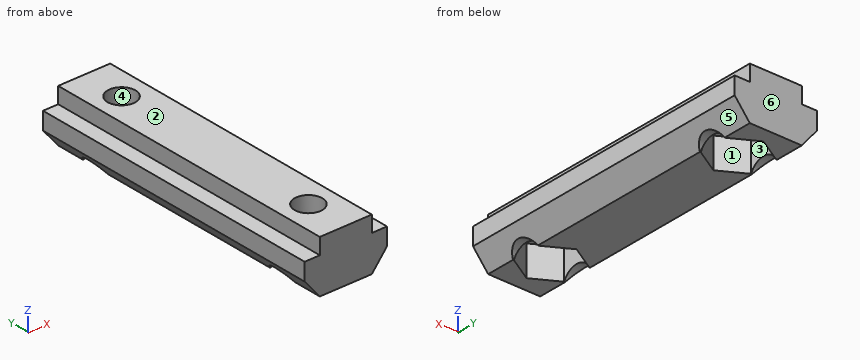
from build123d import *

# Parameters (mm, degrees)
EXTRUDE1_DEPTH = 35
EXTRUDE2_REACH = 8
SKETCH2_R      = 1.6
SKETCH_R       = 1.6
EXTRUDE3_DEPTH = 3.5
EXTRUDE4_START = -0.967619
EXTRUDE4_DEPTH = 7.735238


with BuildPart() as part:
    # Sketch1 → Extrude1 (new body)
    with BuildSketch(Plane(origin=(0, 0, 0), x_dir=(1, 0, 0), z_dir=(0, 1, 0))):
        Polygon((-3, 2.978553588), (3, 2.978553588), (3, 4.828553588), (4.75, 4.828553588), (4.75, 6.828553588), (3, 8.978553588), (-3, 8.978553588), (-4.75, 6.828553588), (-4.75, 4.828553588), (-3, 4.828553588), align=None)
    extrude(amount=EXTRUDE1_DEPTH)

    # Sketch2 → Extrude2 (cut, up to next)
    with BuildSketch(Plane(origin=(0, 0, -8.978553588), x_dir=(-1, 0, 0), z_dir=(0, 0, -1)), mode=Mode.PRIVATE) as extrude2_sk1:
        with Locations((0, 30)):
            Circle(SKETCH2_R)
    extrude2_tool1 = extrude(extrude2_sk1.sketch, amount=-EXTRUDE2_REACH, mode=Mode.PRIVATE) & part.part
    add(extrude2_tool1.solids().sort_by_distance((0, 30, -8.978554))[0], mode=Mode.SUBTRACT)
    # Sketch2 → Extrude2 (cut, up to next)
    with BuildSketch(Plane(origin=(0, 0, -8.978553588), x_dir=(-1, 0, 0), z_dir=(0, 0, -1)), mode=Mode.PRIVATE) as extrude2_sk2:
        with Locations((0, 5)):
            Circle(SKETCH2_R)
    extrude2_tool2 = extrude(extrude2_sk2.sketch, amount=-EXTRUDE2_REACH, mode=Mode.PRIVATE) & part.part
    add(extrude2_tool2.solids().sort_by_distance((0, 5, -8.978554))[0], mode=Mode.SUBTRACT)

    # Sketch → Extrude3 (cut)
    with BuildSketch(Plane(origin=(0, 0, -8.978553588), x_dir=(-1, 0, 0), z_dir=(0, 0, -1))):
        Polygon((0, 33.348631561), (-2.9, 31.674315781), (-2.9, 28.325684219), (0, 26.651368439), (2.9, 28.325684219), (2.9, 31.674315781), align=None)
        with Locations((0, 30)):
            Circle(SKETCH_R, mode=Mode.SUBTRACT)
        Polygon((2.9, 3.325684219), (0, 1.651368439), (-2.9, 3.325684219), (-2.9, 6.674315781), (0, 8.348631561), (2.9, 6.674315781), align=None)
        with Locations((0, 5)):
            Circle(SKETCH_R, mode=Mode.SUBTRACT)
    extrude(amount=-EXTRUDE3_DEPTH, mode=Mode.SUBTRACT)

    # Sketch3 → Extrude4 (cut)
    with BuildSketch(Plane(origin=(-2.9, 0, 0), x_dir=(0, 0, -1), z_dir=(1, 0, 0)).offset(EXTRUDE4_START)):
        with BuildLine():
            Line((8.978553588, 31.674315781), (8.978553588, 28.325684219))
            ThreePointArc((8.978553588, 28.325684219), (7.912621815, 30), (8.978553588, 31.674315781))
        make_face()
    extrude4 = extrude(amount=EXTRUDE4_DEPTH, mode=Mode.SUBTRACT)

    # Mirror1: Extrude4 across plane
    add(extrude4.mirror(Plane.ZX.offset(17.5)), mode=Mode.SUBTRACT)


solid = part.part
Part model, mm, in its own coordinate system. Face numbers are marked on the shaded views. A direction names the side the tool comes from. Give positions to 0.01 mm unless a question says otherwise; leave off trailing zeros. Order: outer loops, then holes, each group sorted by start corner. A loop starts at its lowest first (then second) coordinate and runs counter-clockwise, first axis right, second up. Notation, with made-up numbers: (45, -29) - (64, -29) arc R19 ccw to (64, 6) - close; hole circle Ø4 at (8, -36.75). An arc over 180 degrees is marked (long way). Use a Markdown table: item, result.
1) Saw through at B-B on z = -6.5. List the corners of the cut face in (x, y), plus the area to 3 significant figures.
Checked values:
| item | result |
|---|---|
| outline | (-4.75, 0) - (4.75, 0) - (4.75, 35) - (-4.75, 35) - close; hole (-2.9, 3.33) - (0, 1.65) - (2.9, 3.33) - (2.9, 6.67) - (0, 8.35) - (-2.9, 6.67) - close; hole (-2.9, 28.33) - (0, 26.65) - (2.9, 28.33) - (2.9, 31.67) - (0, 33.35) - (-2.9, 31.67) - close |
| area | 274 mm² |
2) Saw through at A-A on y = 25. List the corners of the cut face in (x, z).
Checked values:
| item | result |
|---|---|
| outline | (-4.75, -6.83) - (-3, -8.98) - (3, -8.98) - (4.75, -6.83) - (4.75, -4.83) - (3, -4.83) - (3, -2.98) - (-3, -2.98) - (-3, -4.83) - (-4.75, -4.83) - close |
3) Flat gauge pins, fed straight in: P1, Ø2.5, axis at x = 0, y = 5, coming from the +Z side; P2, Ø0.6, axis at y = 12.5, z = -4, coming from the -X side; P3, Ø1.7, axis at y = 5.5, z = -8, coming from the +X side; P4, Ø0.9, axis at y = 11, z = -4, coming from the +X side. Where does each tip first touch, or does it go through?
Checked values:
| item | result |
|---|---|
| P1 | through |
| P2 | x = -3 |
| P3 | x = 4.49 |
| P4 | x = 3 |
4) Saw through at D-D on x = 2. List the corners of the cut face in (y, z).
Checked values:
| item | result |
|---|---|
| outline | (0, -8.98) - (2.81, -8.98) - (2.81, -5.48) - (7.19, -5.48) - (7.19, -8.98) - (27.81, -8.98) - (27.81, -5.48) - (32.19, -5.48) - (32.19, -8.98) - (35, -8.98) - (35, -2.98) - (0, -2.98) - close |
5) Saw through at C-C on y = 5. List the corners of the cut face in (x, z).
Checked values:
| item | result |
|---|---|
| outline | (-4.75, -6.83) - (-3.87, -7.91) - (-2.9, -7.91) - (-2.9, -5.48) - (-1.6, -5.48) - (-1.6, -2.98) - (-3, -2.98) - (-3, -4.83) - (-4.75, -4.83) - close; (1.6, -5.48) - (2.9, -5.48) - (2.9, -7.91) - (3.87, -7.91) - (4.75, -6.83) - (4.75, -4.83) - (3, -4.83) - (3, -2.98) - (1.6, -2.98) - close |
6) Two-plate mould, pull along X, no slides. Class the marked faces 3, 4, 5 and 6: +X half, -X half, draft (parallel to the pull), parting line (faces both ways), or undercut.
Checked values:
| item | result |
|---|---|
| face 3 | undercut |
| face 4 | undercut |
| face 5 | +X half |
| face 6 | draft |
7) Probe L1, parallel to Y at x = 0, z = -4.9; L2, parallel to Y at x = -2, z = -7.2; L3, parallel to X at y = 30.5, z = -7.05. List the from-to ranges inside material, lowest first. Write a range as from..to.
Checked values:
| item | result |
|---|---|
| L1 | 0..3.4, 6.6..28.4, 31.6..35 |
| L2 | 0..2.81, 7.19..27.81, 32.19..35 |
| L3 | -4.57..-2.9, 2.9..4.57 |
8) 3-axis set-ups, long thin cutter, end or side, ignore diameter. For the marked faces 1 and 2: which of +Z, -Z, +X, -X, +Y, -Y reach the whole face in a straight line?
Checked values:
| item | result |
|---|---|
| face 1 | -Z |
| face 2 | +Z, +X, -X, +Y, -Y |
